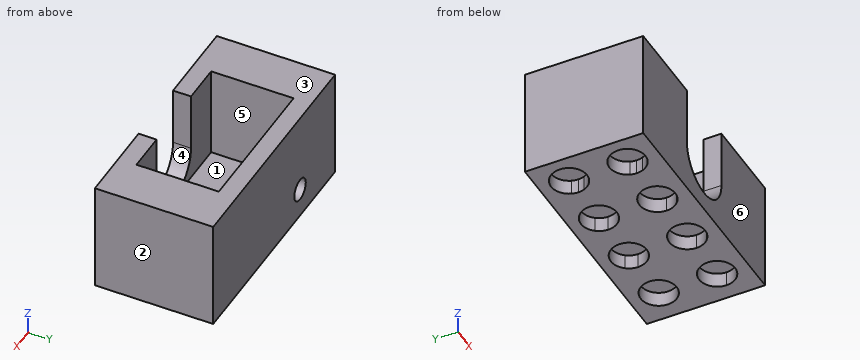
```python
from build123d import *

# Parameters (mm, degrees)
F0_W     = 31.8
F0_H     = 15.8
F1_DEPTH = 15
F3_DEPTH = 2.4
F4_DEPTH = 2.5
F5_R     = 1.5
F6_DEPTH = 2.4
F7_DEPTH = 2


with BuildPart() as f1:
    # F0 (on Top) → F1 (new body)
    with BuildSketch(Plane.XY):
        Rectangle(F0_W, F0_H)
        with BuildLine():
            Line((-9.75, 4.8351646544), (-9.75, 5.5))
            Line((-9.75, 5.5), (-6.0734993995, 5.5))
            ThreePointArc((-6.0734993995, 5.5), (-4.2, 6.4), (-2.3265006005, 5.5))
            Line((-2.3265006005, 5.5), (1.7265006005, 5.5))
            ThreePointArc((1.7265006005, 5.5), (3.6, 6.4), (5.4734993995, 5.5))
            Line((5.4734993995, 5.5), (9.5265006005, 5.5))
            ThreePointArc((9.5265006005, 5.5), (12.1948589312, 6.2645527769), (13.8, 4))
            ThreePointArc((13.8, 4), (12.3486832981, 1.7954592315), (9.75, 2.2571574942))
            Line((9.75, 2.2571574942), (9.75, -2.0571574942))
            ThreePointArc((9.75, -2.0571574942), (12.3486832981, -1.5954592315), (13.8, -3.8))
            ThreePointArc((13.8, -3.8), (12.3203646443, -6.016512784), (9.7058925654, -5.5))
            Line((9.7058925654, -5.5), (5.2941074346, -5.5))
            ThreePointArc((5.2941074346, -5.5), (3.6, -6.2), (1.9058925654, -5.5))
            Line((1.9058925654, -5.5), (-2.5058925654, -5.5))
            ThreePointArc((-2.5058925654, -5.5), (-4.2, -6.2), (-5.8941074346, -5.5))
            Line((-5.8941074346, -5.5), (-9.75, -5.5))
            Line((-9.75, -5.5), (-9.75, -4.6351646544))
            ThreePointArc((-9.75, -4.6351646544), (-14.4, -3.8), (-9.75, -2.9648353456))
            Line((-9.75, -2.9648353456), (-9.75, 3.1648353456))
            ThreePointArc((-9.75, 3.1648353456), (-14.4, 4), (-9.75, 4.8351646544))
        make_face(mode=Mode.SUBTRACT)
        with BuildLine():
            Line((-9.75, -4.6351646544), (-9.75, -2.9648353456))
            ThreePointArc((-9.75, -2.9648353456), (-14.4, -3.8), (-9.75, -4.6351646544))
        make_face()
        with BuildLine():
            Line((-9.75, 3.1648353456), (-9.75, 4.8351646544))
            ThreePointArc((-9.75, 4.8351646544), (-14.4, 4), (-9.75, 3.1648353456))
        make_face()
        with BuildLine():
            ThreePointArc((13.8, 4), (12.1948589312, 6.2645527769), (9.5265006005, 5.5))
            Line((9.5265006005, 5.5), (9.75, 5.5))
            Line((9.75, 5.5), (9.75, 2.2571574942))
            ThreePointArc((9.75, 2.2571574942), (12.3486832981, 1.7954592315), (13.8, 4))
        make_face()
        with BuildLine():
            ThreePointArc((13.8, -3.8), (12.3486832981, -1.5954592315), (9.75, -2.0571574942))
            Line((9.75, -2.0571574942), (9.75, -5.5))
            Line((9.75, -5.5), (9.7058925654, -5.5))
            ThreePointArc((9.7058925654, -5.5), (12.3203646443, -6.016512784), (13.8, -3.8))
        make_face()
        with BuildLine():
            ThreePointArc((-2.3265006005, 5.5), (-4.2, 6.4), (-6.0734993995, 5.5))
            Line((-6.0734993995, 5.5), (-2.3265006005, 5.5))
        make_face()
        with BuildLine():
            ThreePointArc((5.4734993995, 5.5), (3.6, 6.4), (1.7265006005, 5.5))
            Line((1.7265006005, 5.5), (5.4734993995, 5.5))
        make_face()
        with BuildLine():
            Line((5.2941074346, -5.5), (1.9058925654, -5.5))
            ThreePointArc((1.9058925654, -5.5), (3.6, -6.2), (5.2941074346, -5.5))
        make_face()
        with BuildLine():
            Line((-2.5058925654, -5.5), (-5.8941074346, -5.5))
            ThreePointArc((-5.8941074346, -5.5), (-4.2, -6.2), (-2.5058925654, -5.5))
        make_face()
    extrude(amount=F1_DEPTH)

    # F2 (on face) → F3 (cut, through all)
    with BuildSketch(Plane.XZ.offset(7.9)):
        with BuildLine():
            Line((4.5, 15), (-4.5, 15))
            Line((-4.5, 15), (-4.5, 7))
            ThreePointArc((-4.5, 7), (0, 2.5), (4.5, 7))
            Line((4.5, 7), (4.5, 15))
        make_face()
    extrude(amount=-F3_DEPTH, mode=Mode.SUBTRACT)

    # F0 (on Top) → F4 (join)
    with BuildSketch(Plane.XY):
        with BuildLine():
            Line((-6.0734993995, 5.5), (-9.75, 5.5))
            Line((-9.75, 5.5), (-9.75, 4.8351646544))
            ThreePointArc((-9.75, 4.8351646544), (-9.6377976378, 4.4242640687), (-9.6, 4))
            ThreePointArc((-9.6, 4), (-9.6377976378, 3.5757359313), (-9.75, 3.1648353456))
            Line((-9.75, 3.1648353456), (-9.75, -2.9648353456))
            ThreePointArc((-9.75, -2.9648353456), (-9.6377976378, -3.3757359313), (-9.6, -3.8))
            ThreePointArc((-9.6, -3.8), (-9.6377976378, -4.2242640687), (-9.75, -4.6351646544))
            Line((-9.75, -4.6351646544), (-9.75, -5.5))
            Line((-9.75, -5.5), (-5.8941074346, -5.5))
            ThreePointArc((-5.8941074346, -5.5), (-5.1203646443, -1.583487216), (-1.8, -3.8))
            ThreePointArc((-1.8, -3.8), (-1.983487216, -4.7203646443), (-2.5058925654, -5.5))
            Line((-2.5058925654, -5.5), (1.9058925654, -5.5))
            ThreePointArc((1.9058925654, -5.5), (2.6796353557, -1.583487216), (6, -3.8))
            ThreePointArc((6, -3.8), (5.816512784, -4.7203646443), (5.2941074346, -5.5))
            Line((5.2941074346, -5.5), (9.7058925654, -5.5))
            ThreePointArc((9.7058925654, -5.5), (9.0001969324, -3.7692553009), (9.75, -2.0571574942))
            Line((9.75, -2.0571574942), (9.75, 2.2571574942))
            ThreePointArc((9.75, 2.2571574942), (9.0056798702, 3.8349814676), (9.5265006005, 5.5))
            Line((9.5265006005, 5.5), (5.4734993995, 5.5))
            ThreePointArc((5.4734993995, 5.5), (5.8645527769, 4.7948589312), (6, 4))
            ThreePointArc((6, 4), (2.8051410688, 1.7354472231), (1.7265006005, 5.5))
            Line((1.7265006005, 5.5), (-2.3265006005, 5.5))
            ThreePointArc((-2.3265006005, 5.5), (-1.9354472231, 4.7948589312), (-1.8, 4))
            ThreePointArc((-1.8, 4), (-4.9948589312, 1.7354472231), (-6.0734993995, 5.5))
        make_face()
        with BuildLine():
            ThreePointArc((6, -3.8), (2.6796353557, -1.583487216), (1.9058925654, -5.5))
            Line((1.9058925654, -5.5), (5.2941074346, -5.5))
            ThreePointArc((5.2941074346, -5.5), (5.816512784, -4.7203646443), (6, -3.8))
        make_face()
        with BuildLine():
            ThreePointArc((-1.8, -3.8), (-5.1203646443, -1.583487216), (-5.8941074346, -5.5))
            Line((-5.8941074346, -5.5), (-2.5058925654, -5.5))
            ThreePointArc((-2.5058925654, -5.5), (-1.983487216, -4.7203646443), (-1.8, -3.8))
        make_face()
        with BuildLine():
            Line((-2.3265006005, 5.5), (-6.0734993995, 5.5))
            ThreePointArc((-6.0734993995, 5.5), (-4.9948589312, 1.7354472231), (-1.8, 4))
            ThreePointArc((-1.8, 4), (-1.9354472231, 4.7948589312), (-2.3265006005, 5.5))
        make_face()
        with BuildLine():
            Line((5.4734993995, 5.5), (1.7265006005, 5.5))
            ThreePointArc((1.7265006005, 5.5), (2.8051410688, 1.7354472231), (6, 4))
            ThreePointArc((6, 4), (5.8645527769, 4.7948589312), (5.4734993995, 5.5))
        make_face()
        with BuildLine():
            Line((9.75, -5.5), (9.75, -2.0571574942))
            ThreePointArc((9.75, -2.0571574942), (9.0001969324, -3.7692553009), (9.7058925654, -5.5))
            Line((9.7058925654, -5.5), (9.75, -5.5))
        make_face()
        with BuildLine():
            Line((9.75, 5.5), (9.5265006005, 5.5))
            ThreePointArc((9.5265006005, 5.5), (9.0056798702, 3.8349814676), (9.75, 2.2571574942))
            Line((9.75, 2.2571574942), (9.75, 5.5))
        make_face()
        with BuildLine():
            ThreePointArc((-9.6, 4), (-9.6377976378, 4.4242640687), (-9.75, 4.8351646544))
            Line((-9.75, 4.8351646544), (-9.75, 3.1648353456))
            ThreePointArc((-9.75, 3.1648353456), (-9.6377976378, 3.5757359313), (-9.6, 4))
        make_face()
        with BuildLine():
            ThreePointArc((-9.6, -3.8), (-9.6377976378, -3.3757359313), (-9.75, -2.9648353456))
            Line((-9.75, -2.9648353456), (-9.75, -4.6351646544))
            ThreePointArc((-9.75, -4.6351646544), (-9.6377976378, -4.2242640687), (-9.6, -3.8))
        make_face()
    extrude(amount=F4_DEPTH)

    # F5 (on face) → F6 (cut, through all)
    with BuildSketch(Plane(origin=(0, 7.9, 0), x_dir=(-1, 0, 0), z_dir=(0, 1, 0))):
        with Locations((6.75, 4)):
            Circle(F5_R)
    extrude(amount=-F6_DEPTH, mode=Mode.SUBTRACT)

    # F0 (on Top) → F7 (cut)
    with BuildSketch(Plane.XY):
        with BuildLine():
            ThreePointArc((13.8, 4), (12.1948589312, 6.2645527769), (9.5265006005, 5.5))
            Line((9.5265006005, 5.5), (9.75, 5.5))
            Line((9.75, 5.5), (9.75, 2.2571574942))
            ThreePointArc((9.75, 2.2571574942), (12.3486832981, 1.7954592315), (13.8, 4))
        make_face()
        with BuildLine():
            Line((9.75, 5.5), (9.5265006005, 5.5))
            ThreePointArc((9.5265006005, 5.5), (9.0056798702, 3.8349814676), (9.75, 2.2571574942))
            Line((9.75, 2.2571574942), (9.75, 5.5))
        make_face()
        with BuildLine():
            Line((5.4734993995, 5.5), (1.7265006005, 5.5))
            ThreePointArc((1.7265006005, 5.5), (2.8051410688, 1.7354472231), (6, 4))
            ThreePointArc((6, 4), (5.8645527769, 4.7948589312), (5.4734993995, 5.5))
        make_face()
        with BuildLine():
            ThreePointArc((5.4734993995, 5.5), (3.6, 6.4), (1.7265006005, 5.5))
            Line((1.7265006005, 5.5), (5.4734993995, 5.5))
        make_face()
        with BuildLine():
            Line((-2.3265006005, 5.5), (-6.0734993995, 5.5))
            ThreePointArc((-6.0734993995, 5.5), (-4.9948589312, 1.7354472231), (-1.8, 4))
            ThreePointArc((-1.8, 4), (-1.9354472231, 4.7948589312), (-2.3265006005, 5.5))
        make_face()
        with BuildLine():
            ThreePointArc((-2.3265006005, 5.5), (-4.2, 6.4), (-6.0734993995, 5.5))
            Line((-6.0734993995, 5.5), (-2.3265006005, 5.5))
        make_face()
        with BuildLine():
            Line((-9.75, 3.1648353456), (-9.75, 4.8351646544))
            ThreePointArc((-9.75, 4.8351646544), (-14.4, 4), (-9.75, 3.1648353456))
        make_face()
        with BuildLine():
            ThreePointArc((-9.6, 4), (-9.6377976378, 4.4242640687), (-9.75, 4.8351646544))
            Line((-9.75, 4.8351646544), (-9.75, 3.1648353456))
            ThreePointArc((-9.75, 3.1648353456), (-9.6377976378, 3.5757359313), (-9.6, 4))
        make_face()
        with BuildLine():
            Line((-9.75, -4.6351646544), (-9.75, -2.9648353456))
            ThreePointArc((-9.75, -2.9648353456), (-14.4, -3.8), (-9.75, -4.6351646544))
        make_face()
        with BuildLine():
            ThreePointArc((-9.6, -3.8), (-9.6377976378, -3.3757359313), (-9.75, -2.9648353456))
            Line((-9.75, -2.9648353456), (-9.75, -4.6351646544))
            ThreePointArc((-9.75, -4.6351646544), (-9.6377976378, -4.2242640687), (-9.6, -3.8))
        make_face()
        with BuildLine():
            ThreePointArc((-1.8, -3.8), (-5.1203646443, -1.583487216), (-5.8941074346, -5.5))
            Line((-5.8941074346, -5.5), (-2.5058925654, -5.5))
            ThreePointArc((-2.5058925654, -5.5), (-1.983487216, -4.7203646443), (-1.8, -3.8))
        make_face()
        with BuildLine():
            Line((-2.5058925654, -5.5), (-5.8941074346, -5.5))
            ThreePointArc((-5.8941074346, -5.5), (-4.2, -6.2), (-2.5058925654, -5.5))
        make_face()
        with BuildLine():
            ThreePointArc((6, -3.8), (2.6796353557, -1.583487216), (1.9058925654, -5.5))
            Line((1.9058925654, -5.5), (5.2941074346, -5.5))
            ThreePointArc((5.2941074346, -5.5), (5.816512784, -4.7203646443), (6, -3.8))
        make_face()
        with BuildLine():
            Line((5.2941074346, -5.5), (1.9058925654, -5.5))
            ThreePointArc((1.9058925654, -5.5), (3.6, -6.2), (5.2941074346, -5.5))
        make_face()
        with BuildLine():
            ThreePointArc((13.8, -3.8), (12.3486832981, -1.5954592315), (9.75, -2.0571574942))
            Line((9.75, -2.0571574942), (9.75, -5.5))
            Line((9.75, -5.5), (9.7058925654, -5.5))
            ThreePointArc((9.7058925654, -5.5), (12.3203646443, -6.016512784), (13.8, -3.8))
        make_face()
        with BuildLine():
            Line((9.75, -5.5), (9.75, -2.0571574942))
            ThreePointArc((9.75, -2.0571574942), (9.0001969324, -3.7692553009), (9.7058925654, -5.5))
            Line((9.7058925654, -5.5), (9.75, -5.5))
        make_face()
    extrude(amount=F7_DEPTH, mode=Mode.SUBTRACT)


solid = f1.part
```
Part model, mm, in its own coordinate system. Face numbers are marked on the shaded views. A direction names the side the tool comes from. Coordinates: 2 decimals unless noted, no trailing zeros. Order: outer loops, then holes, each group sorted by start corner. A loop starts at its lowest first (then second) coordinate and runs counter-clockwise, first axis right, second up. Notation, with made-up numbers: (79, -26.75) - (130, -26.75) arc R24 ccw to (130, -13.75) - close; hole circle Ø10 at (25.25, 34). An arc over 180 degrees is marked (long way). Return JSON: item names as keys, results as strings. Group by question number.
Item 1: Drill centre lines: probe 1 along X at (y, z) = (-3.8, 1.6); probe 2 along Y at (x, z) = (-12, 0.5); probe 3 along Z at (x, y) = (-6.75, 6.4). Where is each one in solid material? Low to high. Write a range as from..to.
Item 2: Which spindle directions (+Z, -Z, +X, -X, +Y, -Y) get a long thin tool onto all of the face, cutting with end or side? Do the marked faces 4, 5 and 6. Say none if no direction does.
Item 3: Pull direction X, two halves, no side cores. Call the marked faces 1, 2 and 3: pulls with the +X half, pulls with the -X half, needs draft (parallel to the pull), parting line crosses it, or undercut.
Item 4: Cut at D-D (x = 11.4). List the corners of the cut face in (y, z).
Item 5: Cut at A-A (x = 3.6). List the corners of the cut face in (y, z), plus the area to 3 significant figures.
Item 6: Cut at C-C (z = 4). List the corners of the cut face in (x, y), plus the area to 3 significant figures.
Item 7: Cut at B-B (z = 12.25). List the corners of the cut face in (x, y), plus the area to 3 significant figures.
Item 8: Pin check, flat tips, straight feed: pin 1 (6 mm diameter, centred on x = -1, z = 6, fed in from -Y); pin 2 (4 mm diameter, centred on x = -12, y = -3.8, fed in from -Z). Stop position of each tip, or through.
Check values:
{
 "1": {"probe 1": "x = -15.9..-14.4, -9.6..-6.6, -1.8..1.2, 6..9, 13.8..15.9", "probe 2": "y = -7.9..-6.2, -1.4..1.6, 6.4..7.9", "probe 3": "z = 0..2.5, 5.5..15"},
 "2": {"face 4": "+Z, -Y", "face 5": "+Z", "face 6": "+Z, -Z, +X, -X, -Y"},
 "3": {"face 1": "undercut", "face 2": "pulls with the +X half", "face 3": "needs draft"},
 "4": {"outline": "(-7.9, 0) - (-6.2, 0) - (-6.2, 2) - (-1.4, 2) - (-1.4, 0) - (1.6, 0) - (1.6, 2) - (6.4, 2) - (6.4, 0) - (7.9, 0) - (7.9, 15) - (-7.9, 15) - close"},
 "5": {"outline": "(-7.9, 0) - (-6.2, 0) - (-6.2, 2) - (-1.4, 2) - (-1.4, 0) - (1.6, 0) - (1.6, 2) - (6.4, 2) - (6.4, 0) - (7.9, 0) - (7.9, 15) - (5.5, 15) - (5.5, 2.5) - (-5.5, 2.5) - (-5.5, 4.3) - (-7.9, 4.3) - close", "area": "54.6 mm2"},
 "6": {"outline": "(-15.9, -7.9) - (-3.35, -7.9) - (-3.35, -5.5) - (-9.75, -5.5) - (-9.75, 5.5) - (-8.25, 5.5) - (-8.25, 7.9) - (-15.9, 7.9) - close; (-5.25, 5.5) - (9.75, 5.5) - (9.75, -5.5) - (3.35, -5.5) - (3.35, -7.9) - (15.9, -7.9) - (15.9, 7.9) - (-5.25, 7.9) - close", "area": "265 mm2"},
 "7": {"outline": "(-15.9, -7.9) - (-4.5, -7.9) - (-4.5, -5.5) - (-9.75, -5.5) - (-9.75, 5.5) - (9.75, 5.5) - (9.75, -5.5) - (4.5, -5.5) - (4.5, -7.9) - (15.9, -7.9) - (15.9, 7.9) - (-15.9, 7.9) - close", "area": "266 mm2"},
 "8": {"pin 1": "stops at y = 5.5", "pin 2": "stops at z = 2"}
}
